```python
from build123d import *

# Parameters (mm, degrees)
CROQUIS1_R              = 40
SALIENTE_EXTRUIR1_DEPTH = 80
CROQUIS2_R              = 6.35
SALIENTE_EXTRUIR2_DEPTH = 50.8
CROQUIS3_R              = 12.7
SALIENTE_EXTRUIR3_DEPTH = 12.7
SALIENTE_EXTRUIR4_DEPTH = 12.7


with BuildPart() as part:
    # Croquis1 → Saliente-Extruir1 (new body)
    with BuildSketch(Plane(origin=(0, 0, 0), x_dir=(0, 0, -1), z_dir=(1, 0, 0))):
        Circle(CROQUIS1_R)
    extrude(amount=SALIENTE_EXTRUIR1_DEPTH)

    # Croquis2 → Saliente-Extruir2 (add)
    with BuildSketch(Plane(origin=(80, 0, 0), x_dir=(0, 0, -1), z_dir=(1, 0, 0))):
        Circle(CROQUIS2_R)
    extrude(amount=SALIENTE_EXTRUIR2_DEPTH)

    # Croquis3 → Saliente-Extruir3 (add)
    with BuildSketch(Plane(origin=(130.8, 0, 0), x_dir=(0, 0, -1), z_dir=(1, 0, 0))):
        Circle(CROQUIS3_R)
    extrude(amount=SALIENTE_EXTRUIR3_DEPTH)

    # Croquis4 → Saliente-Extruir4 (add)
    with BuildSketch(Plane.ZY.offset(-130.8)):
        with BuildLine():
            Line((11.483957814, -5.422980079), (107.428083159, 146.742000736))
            ThreePointArc((107.428083159, 146.742000736), (0, 341.478305247), (-107.428083159, 146.742000736))
            Line((-107.428083159, 146.742000736), (-11.483957814, -5.422980079))
            ThreePointArc((-11.483957814, -5.422980079), (0, -12.7), (11.483957814, -5.422980079))
        make_face()
        with BuildLine():
            Line((12.567527858, -1.829547361), (98.098634635, 133.820646696))
            ThreePointArc((98.098634635, 133.820646696), (0, 87.478305247), (-98.098634635, 133.820646696))
            Line((-98.098634635, 133.820646696), (-12.567527858, -1.829547361))
            ThreePointArc((-12.567527858, -1.829547361), (0, 12.7), (12.567527858, -1.829547361))
        make_face(mode=Mode.SUBTRACT)
    extrude(amount=-SALIENTE_EXTRUIR4_DEPTH)


solid = part.part
```
For this review, take the finished solid that the model builds, in its own axes (mm). A direction names the side the tool comes from. Give positions to 0.01 mm unless a question says otherwise; leave off trailing zeros. Write each loop counter-clockwise with the first axis right and the second up, starting at its lowest first coordinate (ties: lowest second). Pieces come first, ordered by that corner, then holes.
Item 1: Wall thickness on probe 1 along X at (y, z) = (170, 114); probe 2 along Y at (x, z) = (137.5, 8); probe 3 along Y at (x, z) = (26, 33): over which ranges is each line inside the solid? List them lowest first.
Item 2: Take a section at D-D (x = 97). Give the boundary of the cut face in (y, z), and give its area (3 significant figures).
Item 3: Insertion check: P1, Ø10, axis at x = 110.5, y = 0, coming from the -Z side. The pin has a flat end and moves straight along its axis. Give the tip position at first contact, or say it passes through.
Item 4: Take a section at A-A (z = 0). Give the boundary of the cut face in (x, y).
Item 5: Machinability: for faces 4 (the face through (137.06, 69.59, 58.78)), 5 (the face through (105.04, -6.2, 1.38)), 6 (the face through (137.061, 71.725, -60.128)), which of the approach directions +Z, -Z, +X, -X, +Y, -Y give a long, thin tool a straight path to every point of the face, cutting with its end or side? Answer none if there is none.
Item 6: The part is to be moulded in two halves that separate along Y. For faces 1 (the face through (39.44, -39.05, 8.67)), 2 (the face through (137.06, 87.49, 1.57)), 3 (the face through (137.1, -12.7, -0.2)), say which applies: +Y half, -Y half, draft (parallel to the pull), parting line (faces both ways), or undercut.
Item 7: Take a section at B-B (z = 35.5). Give the boundary of the cut face in (x, y).
Item 8: Take a section at C-C (y = 116). Give the boundary of the cut face in (x, z), and give its area (3 significant figures).
Established:
1. probe 1: x = 130.8 to 143.5
1. probe 2: y = -9.86 to 9.86, 87.73 to 341.23
1. probe 3: y = -22.61 to 22.61
2. outline: circle Ø12.7 at (0, 0)
2. area: 127 mm2
3. P1: stops at z = -6.35
4. outline: (0, -40) - (80, -40) - (80, -6.35) - (130.8, -6.35) - (130.8, -12.7) - (143.5, -12.7) - (143.5, 12.7) - (130.8, 12.7) - (130.8, 6.35) - (80, 6.35) - (80, 40) - (0, 40) - close; (130.8, 87.48) - (143.5, 87.48) - (143.5, 341.48) - (130.8, 341.48) - close
5. face 4: +Z, +X, -Y
5. face 5: none
5. face 6: -Z, +X, -Y
6. face 1: parting line
6. face 2: undercut
6. face 3: -Y half
7. outline: (0, -18.43) - (80, -18.43) - (80, 18.43) - (0, 18.43) - close; (130.8, 32.67) - (143.5, 32.67) - (143.5, 34.54) - (130.8, 34.54) - close; (130.8, 92.54) - (143.5, 92.54) - (143.5, 336.42) - (130.8, 336.42) - close
8. outline: (130.8, -88.04) - (143.5, -88.04) - (143.5, -86.86) - (130.8, -86.86) - close; (130.8, -80.19) - (143.5, -80.19) - (143.5, 80.19) - (130.8, 80.19) - close; (130.8, 86.86) - (143.5, 86.86) - (143.5, 88.04) - (130.8, 88.04) - close
8. area: 2,070 mm2
